Work out the finished part from the listing and answer in its coordinate system (mm). Face numbers are marked on the shaded views. Give positions to 0.01 mm unless a question says otherwise; leave off trailing zeros. Order: outer loops, then holes, each group sorted by start corner. A loop starts at its lowest first (then second) coordinate and runs counter-clockwise, first axis right, second up. Notation, with made-up numbers: (22, -34.75) - (80, -34.75) arc R25 cw to (80, -6.75) - close; hole circle Ø5 at (79.25, 7.25). An arc over 180 degrees is marked (long way). Return JSON: item names as keys, results as strings. Group by question number.
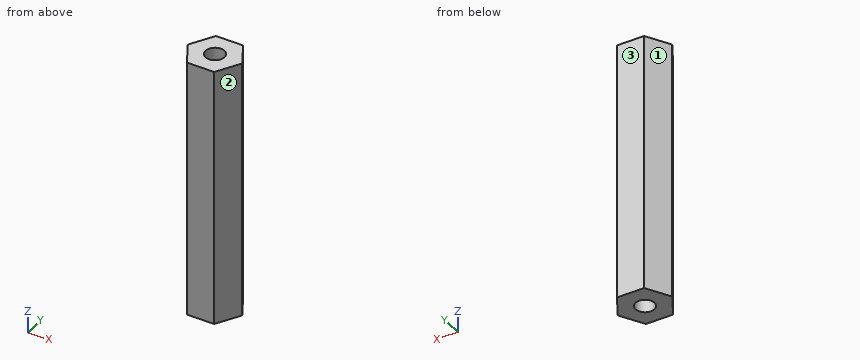
Autodesk Inventor part; units mm, degrees
ref_plane "YZ Plane" through (0, 0, 0) normal (1, 0, 0) x (0, 1, 0)
ref_plane "XZ Plane" through (0, 0, 0) normal (0, 1, 0) x (-1, 0, 0)
ref_plane "XY Plane" through (0, 0, 0) normal (0, 0, 1) x (1, 0, 0)
sketch "Sketch1" plane through (0, 0, 0) normal (0, 0, 1) x (1, 0, 0)
  line L0 (-7.3323, 0) -> (-3.6662, 6.35)
  line L1 (-3.6662, 6.35) -> (3.6662, 6.35)
  line L2 (3.6662, 6.35) -> (7.3323, 0)
  line L3 (7.3323, 0) -> (3.6662, -6.35)
  line L4 (3.6662, -6.35) -> (-3.6662, -6.35)
  line L5 (-3.6662, -6.35) -> (-7.3323, 0)
  circle A0 centre (0, 0) radius 2.5527
  dimension "d0" = 12.7
  dimension "d1" = 5.1054
extrude "Extrusion1" add sketch "Sketch1" along normal blind 70.0024
thread "Thread1"
properties part number "2.756_hexshaft" material "Aluminum 6061"
1. The part is cut by section D-D (y = 5.5). Give the vertices of the cut face in (x, z), and give its area (3 significant figures).
2. The part is cut by section C-C (x = -6.25). Give the vertices of the cut face in (y, z).
3. Each of these flat-tipped pins is pushed along its axis until it touches: pin 1 (6 mm diameter, centred on y = -1, z = 34, fed in from +X); pin 2 (1 mm diameter, centred on x = 0, y = 2, fed in from -Z); pin 3 (1 mm diameter, centred on y = -1, z = 26.5, fed in from +X). Where does it stop, or does it pass through?
4. Consider probe 1 along Y at (x, z) = (0, 39); probe 2 along Y at (x, z) = (-0.25, 19); probe 3 along X at (y, z) = (4.5, 44). Determine where each line is inside the solid, lowest interval first. Write a range as from..to.
5. The part is cut by section A-A (x = 0). Give the vertices of the cut face in (y, z).
6. The part is cut by section B-B (z = 5). Give the vertices of the cut face in (x, y), and give its area (3 significant figures).
7. Determine the mould class of the marked faces 1, 2 and 3 for opening direction X: released by +X, released by -X, zero draft, split by the parting line, or undercut.
Answers:
{
 "1": {"outline": "(-4.16, 0) - (4.16, 0) - (4.16, 70) - (-4.16, 70) - close", "area": "582 mm^2"},
 "2": {"outline": "(-1.87, 0) - (1.87, 0) - (1.87, 70) - (-1.87, 70) - close"},
 "3": {"pin 1": "stops at x = 7.33", "pin 2": "passes through", "pin 3": "stops at x = 7.04"},
 "4": {"probe 1": "y = -6.35..-2.55, 2.55..6.35", "probe 2": "y = -6.35..-2.54, 2.54..6.35", "probe 3": "x = -4.73..4.73"},
 "5": {"outline": "(-6.35, 0) - (-2.55, 0) - (-2.55, 70) - (-6.35, 70) - close; (2.55, 0) - (6.35, 0) - (6.35, 70) - (2.55, 70) - close"},
 "6": {"outline": "(-7.33, 0) - (-3.67, -6.35) - (3.67, -6.35) - (7.33, 0) - (3.67, 6.35) - (-3.67, 6.35) - close; hole circle Ø5.11 at (0, 0)", "area": "119 mm^2"},
 "7": {"face 1": "released by -X", "face 2": "released by +X", "face 3": "zero draft"}
}
